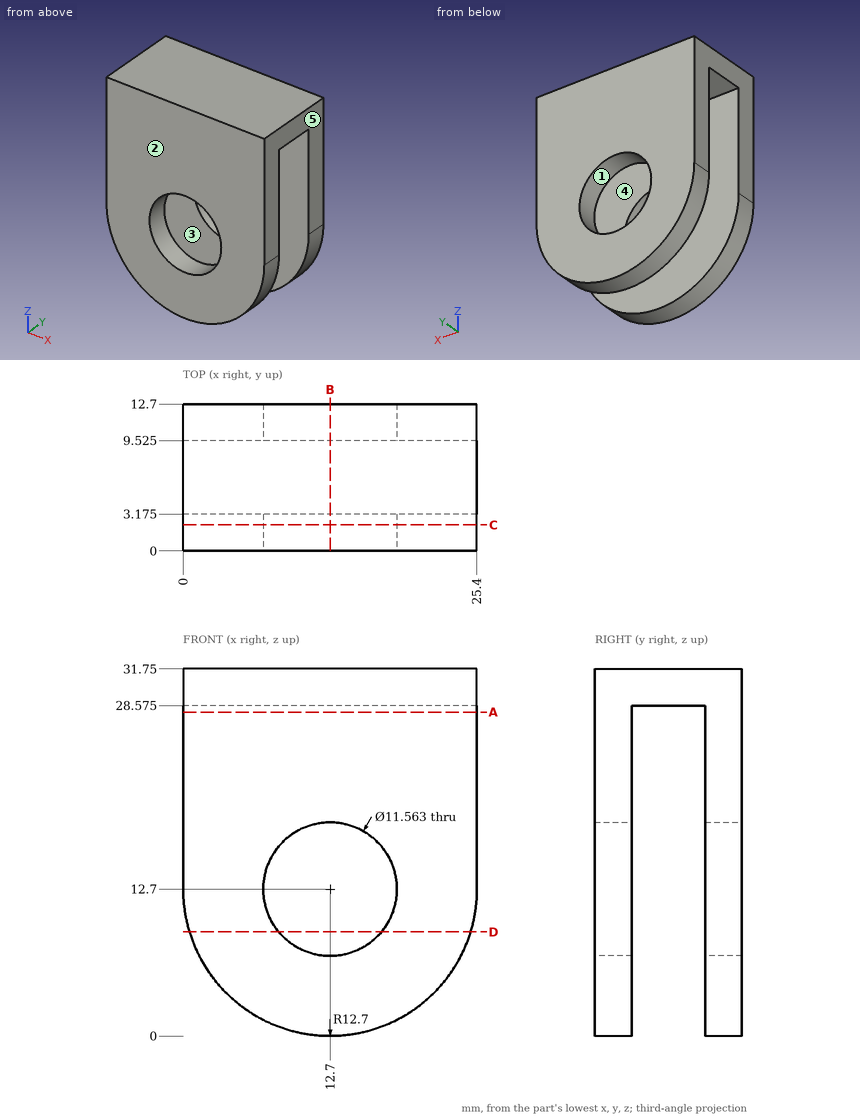
Design review of the part shown in the three views and the two pictorial views. Dimensions are in mm from the part's minimum x, y and z. A direction names the side the tool comes from. Coordinates: 2 decimals unless noted, no trailing zeros. Order: outer loops, then holes, each group sorted by start corner. A loop starts at its lowest first (then second) coordinate and runs counter-clockwise, first axis right, second up.
1) Take a section at B-B, the plane x = 12.7. State how many separate pieces and enclosed holes the cut face has, and give its area (3 significant figures).
2) Clearance check with a flat-ended pin moving along its axis: pin 1 (4 mm diameter, centred on x = 5.5, y = 6.5, fed in from -Z) (3 decimals). State where the tip first meets the part, or that it passes through.
3) Take a section at A-A, the plane z = 28. Give the boundary of the cut face in (x, y) (1 decimal).
4) Take a section at D-D, the plane z = 9. Give the boundary of the cut face in (x, y) (1 decimal).
5) Mouldability with a two-part tool opening along Y and no side actions: class the marked faces 1, 2 and 3 as +Y half, -Y half, draft (parallel to the pull), parting line (faces both ways), or undercut.
6) Wall thickness on line 1 along X through (y, z) = (1.95, 12.7); line 2 along Y through (x, z) = (24.25, 18.5) (1 decimal); line 3 along X through (y, z) = (2.5, 15.5): over which ranges is each line inside the solid? List them lowest first.
7) Take a section at C-C, the plane y = 2.25. Give the boundary of the cut face in (x, z), and give its area (3 significant figures).
8) For the marked faces 4 and 5, list the 3-axis set-ups (+Z, -Z, +X, -X, +Y, -Y) from which the entire face can be reached by the end or side of a thin tool; tool diameter is ignored.
Returned:
1. separate pieces: 3
1. enclosed holes: 0
1. area: 148 mm2
2. pin 1: stops at z = 28.575
3. outline: (0, 0) - (25.4, 0) - (25.4, 3.2) - (0, 3.2) - close; (0, 9.5) - (25.4, 9.5) - (25.4, 12.7) - (0, 12.7) - close
4. outline: (0.6, 0) - (8.3, 0) - (8.3, 3.2) - (0.6, 3.2) - close; (0.6, 9.5) - (8.3, 9.5) - (8.3, 12.7) - (0.6, 12.7) - close; (17.1, 0) - (24.8, 0) - (24.8, 3.2) - (17.1, 3.2) - close; (17.1, 9.5) - (24.8, 9.5) - (24.8, 12.7) - (17.1, 12.7) - close
5. face 1: draft
5. face 2: -Y half
5. face 3: undercut
6. line 1: x = 0 to 6.92, 18.48 to 25.4
6. line 2: y = 0 to 3.2, 9.5 to 12.7
6. line 3: x = 0 to 7.64, 17.76 to 25.4
7. outline: (0, 12.7) arc R12.7 ccw to (25.4, 12.7) - (25.4, 31.75) - (0, 31.75) - close; hole circle Ø11.56 at (12.7, 12.7)
7. area: 632 mm2
8. face 4: -Z, +X, -X
8. face 5: +Z, -Z, +X, +Y, -Y
